Autodesk Inventor part; units mm, degrees
ref_plane "YZ Plane" through (0, 0, 0) normal (1, 0, 0) x (0, 1, 0)
ref_plane "XZ Plane" through (0, 0, 0) normal (0, 1, 0) x (-1, 0, 0)
ref_plane "XY Plane" through (0, 0, 0) normal (0, 0, 1) x (1, 0, 0)
sketch "Sketch1" plane through (0, 0, 0) normal (0, 1, 0) x (-1, 0, 0)
  line L0 (18.4951, 35.5107) -> (-6.9049, 35.5107)
  line L1 (-6.9049, 35.5107) -> (-6.9049, -15.2893)
  line L2 (-6.9049, -15.2893) -> (18.4951, -15.2893)
  line L3 (18.4951, -15.2893) -> (18.4951, 35.5107)
  point P0 (0, 0)
  dimension "d0" = 50.8
  dimension "d1" = 25.4
extrude "Extrusion1" add sketch "Sketch1" along normal blind 3.175
sketch "Sketch2" plane through (0, 3.175, 0) normal (0, 1, 0) x (1, 0, 0)
  line L0 (-18.4951, 15.2893) -> (-18.4951, -35.5107)
  line L1 (6.9049, 15.2893) -> (-18.4951, 15.2893)
  point P0 (0, 0)
  point P1 (-5.7951, -22.8107)
  point P2 (-5.7951, 2.5893)
  dimension "d4" = 12.7
  dimension "d5" = 12.7
  dimension "d6" = 25.4
  dimension "d7" = 12.7
hole "Hole1" at (-5.7951, 3.175, 22.8107) at (-5.7951, 3.175, -2.5893) direction (0, -1, 0) diameter 6.35 end through all
sketch "Sketch3" plane through (0, 3.175, 0) normal (0, 1, 0) x (1, 0, 0)
  line L0 (-12.1451, -19.6357) -> (0.5549, -19.6357)
  line L1 (0.5549, -19.6357) -> (0.5549, -0.5857)
  line L2 (0.5549, -0.5857) -> (-12.1451, -0.5857)
  line L3 (-12.1451, -0.5857) -> (-12.1451, -19.6357)
  line L4 (-18.4951, 15.2893) -> (-18.4951, -35.5107)
  line L5 (6.9049, 15.2893) -> (-18.4951, 15.2893)
  line L6 (-18.4951, -35.5107) -> (6.9049, -35.5107)
  point P0 (0, 0)
  dimension "d15" = 12.7
  dimension "d16" = 6.35
  dimension "d17" = 15.875
  dimension "d18" = 15.875
extrude "Extrusion2" add sketch "Sketch3" along normal blind 25.4
sketch "Sketch4" plane through (0.5549, 3.175, 19.6357) normal (1, 0, 0) x (0, 0, -1)
  circle A0 centre (9.525, 15.24) radius 6.35
  line L0 (19.05, 0) -> (19.05, 25.4)
  line L1 (0, 25.4) -> (19.05, 25.4)
  point P0 (19.6357, -3.175)
  dimension "d21" = 9.525
  dimension "d22" = 12.7
  dimension "d23" = 10.16
extrude "Extrusion3" cut sketch "Sketch4" against normal blind 25.4
properties part number "Main Axle notch"
Check sheet for the modelled part. Datum: model origin and axes. Units: mm. A direction names the side the tool comes from. Give positions to 0.01 mm unless a question says otherwise; leave off trailing zeros. Write each loop counter-clockwise with the first axis right and the second up, starting at its lowest first coordinate (ties: lowest second). Pieces come first, ordered by that corner, then holes. Notation, with made-up numbers: M 81.5,64 L 102.5,64 A22 ccw 102.5,76 Z; hole C 30.5,-36.75 d3. An arc over 180 degrees is marked long. Use one line per item in the form item = value.
(1) Section check C-C on z = 18. Record the boundary of the cut face in (x, y) (3 decimals), plus the area to 3 significant figures.
Answer block:
outline = M -18.495,0 L 6.905,0 L 6.905,3.175 L 0.555,3.175 L 0.555,28.575 L -12.145,28.575 L -12.145,3.175 L -18.495,3.175 Z
area = 403 mm2
(2) Draft check along Z on faces 5 (the flat face through (6.905, 2, 10)), 6 (the flat face through (-6, 2, -15.289)), 7 (the cylindrical face through (-3.863, 1.565, 20.291)). Enter one of: pulls with the +Z half, pulls with the -Z half, needs draft (parallel to the pull), parting line crosses it, or undercut.
Answer block:
face_5 = needs draft
face_6 = pulls with the -Z half
face_7 = undercut
(3) Material ranges on line 1 along Z through (x, y) = (-8, 9); line 2 along X through (y, z) = (11.25, 6.5); line 3 along Y through (x, z) = (-14, -6.5) (3 decimals), recorded low to high.
Answer block:
line_1 = 0.59 to 19.64
line_2 = -12.15 to 0.55
line_3 = 0 to 3.175
(4) Section check B-B on x = -9.5. Record the boundary of the cut face in (y, z) (3 decimals).
Answer block:
outline = M 0,-15.289 L 3.175,-15.289 L 3.175,0.586 L 28.575,0.586 L 28.575,19.636 L 3.175,19.636 L 3.175,35.511 L 0,35.511 Z; hole C 18.415,10.111 d12.7
(5) Tool access check on faces 1 (the flat face through (-6, 16, 19.636)), 2 (the flat face through (0.555, 13, 14)), 3 (the flat face through (-6, 16, 0.586)), 4 (the flat face through (-12.145, 13, 6)). Record the directions out of +Z, -Z, +X, -X, +Y, -Y that give a thin tool (end or side, any length) a straight path to the whole face; none if there is none.
Answer block:
face_1 = +Z, +X, -X, +Y
face_2 = +Z, -Z, +X, +Y
face_3 = -Z, +X, -X, +Y
face_4 = +Z, -Z, -X, +Y
(6) Depth check by flat-ended pin: P1, Ø9.5, axis at y = 11.5, z = 13.5, coming from the +X side; P2, Ø16.5, axis at y = 18.42, z = 10.11, coming from the -X side; P3, Ø1, axis at x = -9, y = 12, coming from the +Z side; P4, Ø1, axis at x = -14, y = 12, coming from the +Z side. Enter the tip coordinate at first touch or a pass-through.
Answer block:
P1 = 0.55
P2 = -12.15
P3 = 19.64
P4 = through
(7) Section check D-D on y = 2. Record the boundary of the cut face in (x, z) (3 decimals), plus the area to 3 significant figures.
Answer block:
outline = M -18.495,-15.289 L 6.905,-15.289 L 6.905,35.511 L -18.495,35.511 Z; hole C -5.795,-2.589 d6.35; hole C -5.795,22.811 d6.35
area = 1,230 mm2
(8) Section check A-A on y = 15. Record the boundary of the cut face in (x, z).
Answer block:
outline = M -12.15,0.59 L 0.55,0.59 L 0.55,4.76 L -12.15,4.76 Z; M -12.15,15.46 L 0.55,15.46 L 0.55,19.64 L -12.15,19.64 Z
